from build123d import *

# Parameters (mm, degrees)
SKETCH2_R           = 8
BOSS_EXTRUDE1_DEPTH = 3
SKETCH3_R           = 5
BOSS_EXTRUDE2_DEPTH = 10
BOSS_EXTRUDE3_DEPTH = 25
SKETCH8_R           = 1.35
CUT_EXTRUDE3_DEPTH  = 10
CUT_EXTRUDE5_DEPTH  = 23.5


with BuildPart() as part:
    # Sketch2 → Boss-Extrude1 (new body)
    with BuildSketch(Plane(origin=(0, 0, 0), x_dir=(0, 0, -1), z_dir=(1, 0, 0))):
        Circle(SKETCH2_R)
    extrude(amount=BOSS_EXTRUDE1_DEPTH)

    # Sketch3 → Boss-Extrude2 (add)
    with BuildSketch(Plane(origin=(3, 0, 0), x_dir=(0, 0, -1), z_dir=(1, 0, 0))):
        Circle(SKETCH3_R)
    extrude(amount=BOSS_EXTRUDE2_DEPTH)

    # Sketch6 → Boss-Extrude3 (add)
    with BuildSketch(Plane(origin=(13, 0, 0), x_dir=(0, 0, -1), z_dir=(1, 0, 0))):
        Polygon((2.389986953, -4.286174949), (4.906929868, -0.073298058), (2.516942915, 4.212876891), (-2.389986953, 4.286174949), (-4.906929868, 0.073298058), (-2.516942915, -4.212876891), align=None)
    extrude(amount=BOSS_EXTRUDE3_DEPTH)

    # Sketch8 → Cut-Extrude3 (cut)
    with BuildSketch(Plane(origin=(38, 0, 0), x_dir=(0, 0, -1), z_dir=(1, 0, 0))):
        Circle(SKETCH8_R)
    extrude(amount=-CUT_EXTRUDE3_DEPTH, mode=Mode.SUBTRACT)

    # Sketch5 → Cut-Extrude5 (cut)
    with BuildSketch(Plane.ZY):
        Polygon((0, -2.309401077), (2, -1.154700538), (2, 1.154700538), (0, 2.309401077), (-2, 1.154700538), (-2, -1.154700538), align=None)
    extrude(amount=-CUT_EXTRUDE5_DEPTH, mode=Mode.SUBTRACT)


solid = part.part
Read the model definition and answer for the solid it produces. Units are mm, in the model's axes. A direction names the side the tool comes from. Round coordinates to 2 decimals unless told otherwise and drop trailing zeros. Order: outer loops, then holes, each group sorted by start corner. A loop starts at its lowest first (then second) coordinate and runs counter-clockwise, first axis right, second up.
1) The part is cut by section D-D on z = -3.25. Write down the section's boundary in (x, y), plus the area to 3 significant figures.
2) The part is cut by section C-C on x = 12.5. Write down the section's boundary in (y, z).
3) Straight lines are drawn through the part: L1, parallel to X at y = -4.75, z = -2.25; L2, parallel to X at y = -2.25, z = -4; L3, parallel to Y at x = 31.25, z = 0. For each, find the intervals that lie inside material, in ascending order.
4) The mould has two halves that part along Y. Classify faces 6 (the face through (12, 0, 2)), 7 (the face through (7.93, -4.88, 1.08)), 8 (the face through (25.32, 2.21, 3.63)): released by +Y, released by -Y, zero draft, split by the parting line, or undercut.
5) For faces 1 (the face through (28, 0, 0)), 2 (the face through (11.586, -1.724, -1.014)), 3 (the face through (25.32, 2.04, -3.73)), 4 (the face through (25.32, -2.21, -3.63)), 5 (the face through (1.48, -7.81, 1.73)), determine the directions among +Z, -Z, +X, -X, +Y, -Y from which every point of the face is accessible in a straight line to the end or side of a thin tool.
6) The part is cut by section B-B on x = 24. Write down the section's boundary in (y, z), plus the area to 3 significant figures.
7) The part is cut by section A-A on x = 31.5. Write down the section's boundary in (y, z).
8) Flat-ended cylindrical pins translate along their axes: pin 1 (1.5 mm diameter, centred on x = 23.5, z = 0, fed in from +Y); pin 2 (4 mm diameter, centred on x = 15, z = 5.5, fed in from -Y); pin 3 (6 mm diameter, centred on x = 21, z = -6, fed in from -Y). Find the tip coordinate at first contact, or state that the pin passes through.
Resolved:
1. outline: (0, -7.31) - (3, -7.31) - (3, -3.8) - (13, -3.8) - (13, -2.85) - (38, -2.85) - (38, 2.9) - (13, 2.9) - (13, 3.8) - (3, 3.8) - (3, 7.31) - (0, 7.31) - close
1. area: 263 mm2
2. outline: circle Ø10 at (0, 0); hole (-2.31, 0) - (-1.15, -2) - (1.15, -2) - (2.31, 0) - (1.15, 2) - (-1.15, 2) - close
3. L1: x = 0 to 3
3. L2: x = 0 to 13
3. L3: y = -4.25 to -1.35, 1.35 to 4.25
4. face 6: undercut
4. face 7: split by the parting line
4. face 8: released by +Y
5. face 1: +X
5. face 2: -X
5. face 3: -Z, +X, +Y
5. face 4: -Z, +X, -Y
5. face 5: +X, -X
6. outline: (-4.29, -2.39) - (-0.07, -4.91) - (4.21, -2.52) - (4.29, 2.39) - (0.07, 4.91) - (-4.21, 2.52) - close
6. area: 62.6 mm2
7. outline: (-4.29, -2.39) - (-0.07, -4.91) - (4.21, -2.52) - (4.29, 2.39) - (0.07, 4.91) - (-4.21, 2.52) - close; hole circle Ø2.7 at (0, 0)
8. pin 1: stops at y = 4.26
8. pin 2: stops at y = -2.45
8. pin 3: stops at y = -3.27
